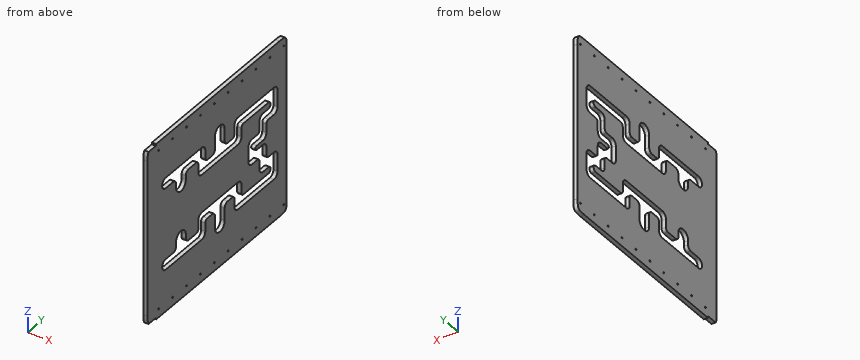
from build123d import *

# Parameters (mm, degrees)
SKETCH_5_W          = 240
SKETCH_5_H          = 480
EXTRUDE_4_DEPTH     = 10
FILLET_1_R          = 7.5
FILLET_2_R          = 5
SKETCH_6_W          = 10
SKETCH_6_H          = 480
EXTRUDE_5_DEPTH     = 90
SKETCH_7_W          = 10
SKETCH_7_H          = 480
EXTRUDE_6_DEPTH     = 90
SKETCH_8_W          = 10
SKETCH_8_H          = 420
EXTRUDE_7_DEPTH     = 20
FILLET_4_SIZE       = 25
SKETCH_9_R          = 1.75
CUT_EXTRUDE_1_DEPTH = 20
SKETCH_10_W         = 4
SKETCH_10_H         = 30
CUT_EXTRUDE_2_DEPTH = 20
FILLET_5_R          = 1
FILLET_6_R          = 1
CUT_EXTRUDE_3_DEPTH = 10
FILLET_7_R          = 10


# Some blends are built 0.0001 mm under size
with BuildPart() as part:
    # 草图5 → 凸台-拉伸4 (new body)
    with BuildSketch(Plane(origin=(0, 0, 0), x_dir=(0, 0, -1), z_dir=(1, 0, 0))):
        Rectangle(SKETCH_5_W, SKETCH_5_H)
        with BuildLine():
            ThreePointArc((-85, -195), (-97.5, -207.5), (-110, -195))
            Line((-110, -195), (-110, -65))
            ThreePointArc((-110, -65), (-106.338834765, -56.161165235), (-97.5, -52.5))
            Line((-97.5, -52.5), (-70, -52.5))
            Line((-70, -52.5), (-70, 52.5))
            Line((-70, 52.5), (-97.5, 52.5))
            ThreePointArc((-97.5, 52.5), (-106.338834765, 56.161165235), (-110, 65))
            Line((-110, 65), (-110, 195))
            ThreePointArc((-110, 195), (-106.338834765, 203.838834765), (-97.5, 207.5))
            Line((-97.5, 207.5), (-57.5, 207.5))
            ThreePointArc((-57.5, 207.5), (-48.661165235, 203.838834765), (-45, 195))
            Line((-45, 195), (-45, 167.5))
            Line((-45, 167.5), (-17.5, 167.5))
            ThreePointArc((-17.5, 167.5), (-8.661165235, 163.838834765), (-5, 155))
            Line((-5, 155), (-5, 127.5))
            Line((-5, 127.5), (5, 127.5))
            Line((5, 127.5), (5, 155))
            ThreePointArc((5, 155), (8.661165235, 163.838834765), (17.5, 167.5))
            Line((17.5, 167.5), (45, 167.5))
            Line((45, 167.5), (45, 195))
            ThreePointArc((45, 195), (48.661165235, 203.838834765), (57.5, 207.5))
            Line((57.5, 207.5), (97.5, 207.5))
            ThreePointArc((97.5, 207.5), (106.338834765, 203.838834765), (110, 195))
            Line((110, 195), (110, 65))
            ThreePointArc((110, 65), (106.338834765, 56.161165235), (97.5, 52.5))
            Line((97.5, 52.5), (70, 52.5))
            Line((70, 52.5), (70, -52.5))
            Line((70, -52.5), (97.5, -52.5))
            ThreePointArc((97.5, -52.5), (106.338834765, -56.161165235), (110, -65))
            Line((110, -65), (110, -195))
            ThreePointArc((110, -195), (97.5, -207.5), (85, -195))
            Line((85, -195), (85, -77.5))
            Line((85, -77.5), (57.5, -77.5))
            ThreePointArc((57.5, -77.5), (48.661165235, -73.838834765), (45, -65))
            Line((45, -65), (45, 65))
            ThreePointArc((45, 65), (48.661165235, 73.838834765), (57.5, 77.5))
            Line((57.5, 77.5), (85, 77.5))
            Line((85, 77.5), (85, 182.5))
            Line((85, 182.5), (70, 182.5))
            Line((70, 182.5), (70, 155))
            ThreePointArc((70, 155), (66.338834765, 146.161165235), (57.5, 142.5))
            Line((57.5, 142.5), (30, 142.5))
            Line((30, 142.5), (30, 115))
            ThreePointArc((30, 115), (26.338834765, 106.161165235), (17.5, 102.5))
            Line((17.5, 102.5), (-17.5, 102.5))
            ThreePointArc((-17.5, 102.5), (-26.338834765, 106.161165235), (-30, 115))
            Line((-30, 115), (-30, 142.5))
            Line((-30, 142.5), (-57.5, 142.5))
            ThreePointArc((-57.5, 142.5), (-66.338834765, 146.161165235), (-70, 155))
            Line((-70, 155), (-70, 182.5))
            Line((-70, 182.5), (-85, 182.5))
            Line((-85, 182.5), (-85, 77.5))
            Line((-85, 77.5), (-57.5, 77.5))
            ThreePointArc((-57.5, 77.5), (-48.661165235, 73.838834765), (-45, 65))
            Line((-45, 65), (-45, -65))
            ThreePointArc((-45, -65), (-48.661165235, -73.838834765), (-57.5, -77.5))
            Line((-57.5, -77.5), (-85, -77.5))
            Line((-85, -77.5), (-85, -195))
        make_face(mode=Mode.SUBTRACT)
    extrude(amount=EXTRUDE_4_DEPTH)

    # 圆角1
    fillet_1_edges = [part.edges().sort_by_distance(p)[0] for p in [
        (5, -77.5, 85),
        (5, -52.5, 70),
        (5, 52.5, 70),
        (5, 77.5, 85),
        (5, 182.5, 85),
        (5, 182.5, 70),
        (5, 167.5, 45),
        (5, 142.5, 30),
        (5, 142.5, -30),
        (5, 167.5, -45),
        (5, 182.5, -70),
        (5, 182.5, -85),
        (5, 77.5, -85),
        (5, 52.5, -70),
        (5, -77.5, -85),
        (5, -52.5, -70),
    ]]
    fillet(fillet_1_edges, radius=FILLET_1_R - 0.0001)  # a hair under: the kernel refuses the full size

    # 圆角2
    fillet_2_edges = [part.edges().sort_by_distance(p)[0] for p in [
        (5, 127.5, 5),
        (5, 127.5, -5),
    ]]
    fillet(fillet_2_edges, radius=FILLET_2_R - 0.0001)  # a hair under: the kernel refuses the full size

    # 草图6 → 凸台-拉伸5 (add)
    with BuildSketch(Plane.XY.offset(120)):
        with Locations((5, 0)):
            Rectangle(SKETCH_6_W, SKETCH_6_H)
    extrude(amount=EXTRUDE_5_DEPTH)

    # 草图7 → 凸台-拉伸6 (add)
    with BuildSketch(Plane(origin=(0, 0, -120), x_dir=(-1, 0, 0), z_dir=(0, 0, -1))):
        with Locations((-5, 0)):
            Rectangle(SKETCH_7_W, SKETCH_7_H)
    extrude(amount=EXTRUDE_6_DEPTH)

    # 草图8 → 凸台-拉伸7 (add)
    with BuildSketch(Plane.XZ.offset(240)):
        with Locations((5, 0)):
            Rectangle(SKETCH_8_W, SKETCH_8_H)
    extrude(amount=EXTRUDE_7_DEPTH)

    # 圆角4
    # a fillet whose section is not a circle: 25 mm, written as the material it takes off along each edge
    with BuildSketch(Plane(origin=(72.5, -260, 210), x_dir=(0, 0, -1), z_dir=(-1, 0, 0)), Plane(origin=(-62.5, 240, -210), x_dir=(0, -1, 0), z_dir=(1, 0, 0)), Plane(origin=(72.5, 240, 210), x_dir=(0, -1, 0), z_dir=(-1, 0, 0))) as fillet_4_piece_1:
        with BuildLine():
            Bezier((FILLET_4_SIZE, 0), (0, 0), (0, -FILLET_4_SIZE), weights=[1, 2.357022604, 1])
            Line((0, -FILLET_4_SIZE), (0, 0))
            Line((0, 0), (FILLET_4_SIZE, 0))
        make_face()
    extrude(amount=135, mode=Mode.SUBTRACT)
    with BuildSketch(Plane(origin=(-62.5, -260, -210), x_dir=(0, 1, 0), z_dir=(1, 0, 0))) as fillet_4_piece_2:
        with BuildLine():
            Bezier((FILLET_4_SIZE, 0), (0, 0), (0, FILLET_4_SIZE), weights=[1, 2.357022604, 1])
            Line((0, FILLET_4_SIZE), (0, 0))
            Line((0, 0), (FILLET_4_SIZE, 0))
        make_face()
    extrude(amount=135, mode=Mode.SUBTRACT)

    # 草图9 → 切除-拉伸1 (cut)
    with BuildSketch(Plane(origin=(10, 0, 0), x_dir=(0, 0, -1), z_dir=(1, 0, 0))):
        with Locations((-190, -220)):
            Circle(SKETCH_9_R)
        with Locations((190, -220)):
            Circle(SKETCH_9_R)
        with Locations((190, -170)):
            Circle(SKETCH_9_R)
        with Locations((190, -120)):
            Circle(SKETCH_9_R)
        with Locations((190, -70)):
            Circle(SKETCH_9_R)
        with Locations((-190, -170)):
            Circle(SKETCH_9_R)
        with Locations((-190, -120)):
            Circle(SKETCH_9_R)
        with Locations((-190, -70)):
            Circle(SKETCH_9_R)
        with Locations((-190, -20)):
            Circle(SKETCH_9_R)
        with Locations((190, -20)):
            Circle(SKETCH_9_R)
        with Locations((-190, 30)):
            Circle(SKETCH_9_R)
        with Locations((190, 30)):
            Circle(SKETCH_9_R)
        with Locations((-190, 80)):
            Circle(SKETCH_9_R)
        with Locations((190, 80)):
            Circle(SKETCH_9_R)
        with Locations((-190, 130)):
            Circle(SKETCH_9_R)
        with Locations((190, 130)):
            Circle(SKETCH_9_R)
        with Locations((-190, 180)):
            Circle(SKETCH_9_R)
        with Locations((190, 180)):
            Circle(SKETCH_9_R)
        with Locations((-190, 230)):
            Circle(SKETCH_9_R)
        with Locations((190, 230)):
            Circle(SKETCH_9_R)
    extrude(amount=-CUT_EXTRUDE_1_DEPTH, mode=Mode.SUBTRACT)

    # 草图10 → 切除-拉伸2 (cut)
    with BuildSketch(Plane(origin=(10, 0, 0), x_dir=(0, 0, -1), z_dir=(1, 0, 0))):
        with Locations((-208, -245)):
            Rectangle(SKETCH_10_W, SKETCH_10_H)
    cut_extrude_2 = extrude(amount=-CUT_EXTRUDE_2_DEPTH, mode=Mode.SUBTRACT)

    # 圆角5
    fillet_5_edges = [part.edges().sort_by_distance(p)[0] for p in [
        (5, -230, 210),
    ]]
    fillet(fillet_5_edges, radius=FILLET_5_R)

    # 镜向2: 切除-拉伸2 across plane
    add(cut_extrude_2.mirror(Plane.XY), mode=Mode.SUBTRACT)

    # 圆角6
    fillet_6_edges = [part.edges().sort_by_distance(p)[0] for p in [
        (5, -230, -210),
    ]]
    fillet(fillet_6_edges, radius=FILLET_6_R)

    # 草图11 → 切除-拉伸3 (cut)
    with BuildSketch(Plane(origin=(10, 0, 0), x_dir=(0, 0, -1), z_dir=(1, 0, 0))):
        with BuildLine():
            Line((-110, -17.5), (-70, -17.5))
            Line((-70, -17.5), (-70, 17.5))
            Line((-70, 17.5), (-110, 17.5))
            ThreePointArc((-110, 17.5), (-127.5, 0), (-110, -17.5))
        make_face()
        with BuildLine():
            Line((110, 17.5), (70, 17.5))
            Line((70, 17.5), (70, -17.5))
            Line((70, -17.5), (110, -17.5))
            ThreePointArc((110, -17.5), (127.5, 0), (110, 17.5))
        make_face()
        with BuildLine():
            Line((85, -157.5), (85, -122.5))
            Line((85, -122.5), (65, -122.5))
            ThreePointArc((65, -122.5), (47.5, -140), (65, -157.5))
            Line((65, -157.5), (85, -157.5))
        make_face()
        with BuildLine():
            Line((-65, -122.5), (-85, -122.5))
            Line((-85, -122.5), (-85, -157.5))
            Line((-85, -157.5), (-65, -157.5))
            ThreePointArc((-65, -157.5), (-47.5, -140), (-65, -122.5))
        make_face()
    extrude(amount=-CUT_EXTRUDE_3_DEPTH, mode=Mode.SUBTRACT)

    # 圆角7
    fillet_7_edges = [part.edges().sort_by_distance(p)[0] for p in [
        (5, -157.5, 85),
        (5, -122.5, 85),
        (5, -122.5, -85),
        (5, -157.5, -85),
        (5, -17.5, -70),
        (5, 17.5, -70),
        (5, 17.5, 70),
        (5, -17.5, 70),
    ]]
    fillet(fillet_7_edges, radius=FILLET_7_R)


solid = part.part
For this review, take the finished solid that the model builds, in its own axes (mm). Round coordinates to 2 decimals unless told otherwise and drop trailing zeros. Loops run counter-clockwise (first coordinate to the right, second up) from the corner with the lowest first, then second, coordinate; pieces in that order, holes last. Notation, with made-up numbers: (46.25, -11.5) - (96.25, -11.5) arc R20 cw to (96.25, 15.5) - close; hole circle Ø2 at (-25.75, 63.5). An arc over 180 degrees is marked (long way). Answer as CSV lines item,"result".
(1) Wall thickness on line 1 (Z direction, x = 8.5, y = -84); line 2 (Z direction, x = 9.5, y = 185); line 3 (Z direction, x = 5.5, y = 80): over which ranges is each line inside the solid? List them lowest first.
Checked values:
line 1,"z = -210 to -110, -84.93 to 84.93, 110 to 210"
line 2,"z = -210 to -110, -45 to 45, 110 to 210"
line 3,"z = -210 to -191.75, -188.25 to -110, -83.09 to 83.09, 110 to 188.25, 191.75 to 210"
(2) Insertion check: P1, Ø4, axis at y = -220, z = 190, coming from the -X side. The pin has a flat end and moves straight along its axis. Give the tip position at first contact, or say it passes through.
Checked values:
P1,"stops at x = 0"
(3) Consider section A-A on x = 2. Give the number of separate pieces and of enclosed holes in the cut face, then the cut area to 3 significant figures.
Checked values:
separate pieces,"1"
enclosed holes,"21"
area,"171,000 mm2"
(4) Consider section B-B on y = 5. Give the boundary of the cut face in (x, z).
Checked values:
outline,"(0, -210) - (10, -210) - (10, -126.77) - (0, -126.77) - close; (0, -45) - (10, -45) - (10, 45) - (0, 45) - close; (0, 126.77) - (10, 126.77) - (10, 210) - (0, 210) - close"
(5) Consider section C-C on y = 149. Give the boundary of the cut face in (x, z), then the cut area to 3 significant figures.
Checked values:
outline,"(0, -210) - (10, -210) - (10, -110) - (0, -110) - close; (0, -85) - (10, -85) - (10, -68.47) - (0, -68.47) - close; (0, -5) - (10, -5) - (10, 5) - (0, 5) - close; (0, 68.47) - (10, 68.47) - (10, 85) - (0, 85) - close; (0, 110) - (10, 110) - (10, 210) - (0, 210) - close"
area,"2,430 mm2"
